Work out the finished part from the listing and answer in its coordinate system (mm). Face numbers are marked on the shaded views. A direction names the side the tool comes from. Round coordinates to 2 decimals unless told otherwise and drop trailing zeros. Loops run counter-clockwise (first coordinate to the right, second up) from the corner with the lowest first, then second, coordinate; pieces in that order, holes last.
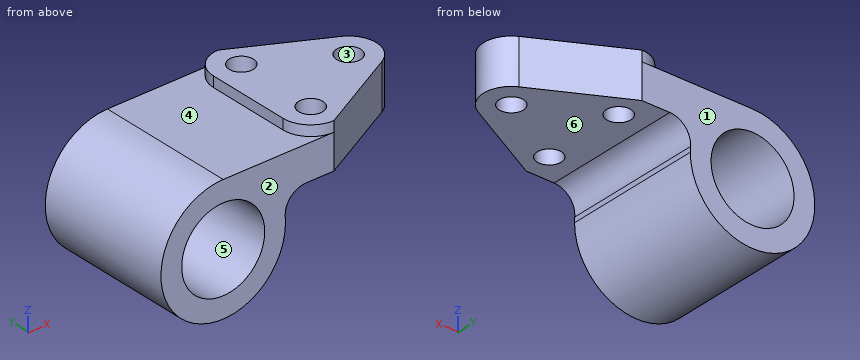
from build123d import *

# Parameters (mm, degrees)
F0_R          = 19.05
F1_DEPTH      = 63.5
F2_R          = 5.5626
F3_DEPTH      = 4.7752
F3_DEPTH_BACK = 15.875
F4_DEPTH      = 57.151


with BuildPart() as f1:
    # F0 (on Front) → F1 (new body)
    with BuildSketch(Plane.XZ):
        with BuildLine():
            ThreePointArc((0, 28.575), (19.345366451, 21.0306305629), (28.4756083945, 2.38125))
            ThreePointArc((28.4756083945, 2.38125), (30.9572676717, 9.6234554837), (37.9674778593, 12.7))
            Line((37.9674778593, 12.7), (50.8, 12.7))
            Line((50.8, 12.7), (50.8, 28.575))
            Line((50.8, 28.575), (0, 28.575))
        make_face()
        with BuildLine():
            ThreePointArc((0, 28.575), (-20.2055762724, -20.2055762724), (28.575, 0))
            ThreePointArc((28.575, 0), (28.5501412858, 1.1916616816), (28.4756083945, 2.38125))
            ThreePointArc((28.4756083945, 2.38125), (19.345366451, 21.0306305629), (0, 28.575))
        make_face()
        Circle(F0_R, mode=Mode.SUBTRACT)
    extrude(amount=F1_DEPTH)

    # F2 (on face) → F3 (join, two sides)
    with BuildSketch(Plane.XY.offset(28.575)) as f3_sk:
        with BuildLine():
            Line((90.0304863666, -20.4933472006), (50.8, 0))
            ThreePointArc((50.8, 0), (41.8197438789, -3.7197438789), (38.1, -12.7))
            Line((38.1, -12.7), (38.1, -50.8))
            ThreePointArc((38.1, -50.8), (41.8197438789, -59.7802561211), (50.8, -63.5))
            Line((50.8, -63.5), (90.0304863666, -43.0066527994))
            ThreePointArc((90.0304863666, -43.0066527994), (96.8502, -31.75), (90.0304863666, -20.4933472006))
        make_face()
        with Locations((50.8, -50.8)):
            Circle(F2_R, mode=Mode.SUBTRACT)
        with Locations((50.8, -12.7)):
            Circle(F2_R, mode=Mode.SUBTRACT)
        with Locations((84.1502, -31.75)):
            Circle(F2_R, mode=Mode.SUBTRACT)
    extrude(amount=F3_DEPTH)
    extrude(f3_sk.sketch, amount=-F3_DEPTH_BACK)

    # F2 (on face) → F4 (cut, through all)
    with BuildSketch(Plane.XY.offset(28.575)):
        with BuildLine():
            Line((50.8, -18.2626), (50.8, -7.1374))
            ThreePointArc((50.8, -7.1374), (45.2374, -12.7), (50.8, -18.2626))
        make_face()
        with BuildLine():
            Line((50.8, -56.3626), (50.8, -45.2374))
            ThreePointArc((50.8, -45.2374), (45.2374, -50.8), (50.8, -56.3626))
        make_face()
    extrude(amount=-F4_DEPTH, mode=Mode.SUBTRACT)


solid = f1.part
Item 1: Section B-B, the plane z = 17.5 is taken. Give the vertices of the cut face in (x, y).
Item 2: Section D-D, the plane z = -4.5 is taken. Give the vertices of the cut face in (x, y), plus the area to 3 significant figures.
Item 3: Section A-A, the plane y = -31.75 is taken. Give the vertices of the cut face in (x, z) (3 decimals).
Item 4: Section C-C, the plane x = 86 is taken. Give the vertices of the cut face in (y, z), plus the area to 3 significant figures.
Item 5: Straight lines are drawn through the part: line 1 (Y direction, x = 50.8, z = 25.5); line 2 (Z direction, x = 1, y = -9) (1 decimal); line 3 (X direction, y = -12.5, z = 1). For each, find the intervals that lie inside material, in ascending order.
Item 6: Each of these flat-tipped pins is pushed along its axis until it touches: P1, Ø2.5, axis at y = -34, z = 31, coming from the -X side; P2, Ø4, axis at y = -30, z = -15, coming from the -X side; P3, Ø3, axis at y = -37, z = -7, coming from the -X side. Where does it stop, or does it pass through?
Item 7: Determine the mould class of the marked faces 1, 2, 3 and 4 for opening direction Y: pulls with the +Y half, pulls with the -Y half, needs draft (parallel to the pull), parting line crosses it, or undercut.
Item 8: For the marked faces 5 and 6, determine the directions among +Z, -Z, +X, -X, +Y, -Y from which every point of the face is accessible in a straight line to the end or side of a thin tool.
Answer below:
1. outline: (-22.59, -63.5) - (-7.53, -63.5) - (-7.53, 0) - (-22.59, 0) - close; (7.53, -63.5) - (50.8, -63.5) - (90.03, -43.01) arc R12.7 ccw to (90.03, -20.49) - (50.8, 0) - (7.53, 0) - close; hole circle Ø11.13 at (50.8, -50.8); hole circle Ø11.13 at (50.8, -12.7); hole circle Ø11.13 at (84.15, -31.75)
2. outline: (-28.22, -63.5) - (-18.51, -63.5) - (-18.51, 0) - (-28.22, 0) - close; (18.51, -63.5) - (28.22, -63.5) - (28.22, 0) - (18.51, 0) - close
2. area: 1,230 mm2
3. outline: (0, 28.575) arc R28.575 ccw (long way) to (28.476, 2.381) arc R9.525 cw to (37.967, 12.7) - (78.588, 12.7) - (78.588, 33.35) - (38.1, 33.35) - (38.1, 28.575) - close; (89.713, 12.7) - (96.85, 12.7) - (96.85, 33.35) - (89.713, 33.35) - close; hole circle Ø38.1 at (0, 0)
4. outline: (-45.11, 12.7) - (-37, 12.7) - (-37, 33.35) - (-45.11, 33.35) - close; (-26.5, 12.7) - (-18.39, 12.7) - (-18.39, 33.35) - (-26.5, 33.35) - close
4. area: 335 mm2
5. line 1: y = -63.5 to -56.36, -45.24 to -18.26, -7.14 to 0
5. line 2: z = -28.6 to -19, 19 to 28.6
5. line 3: x = -28.56 to -19.02, 19.02 to 28.56
6. P1: stops at x = 38.1
6. P2: stops at x = -25.45
6. P3: stops at x = -28.04
7. face 1: pulls with the +Y half
7. face 2: pulls with the -Y half
7. face 3: undercut
7. face 4: needs draft
8. face 5: +Y, -Y
8. face 6: -Z, +X, +Y, -Y
